```python
from build123d import *

# Parameters (mm, degrees)
SKETCH1_W               = 11.9
SKETCH1_H               = 11.9
BOSS_EXTRUDE1_DEPTH     = 3
CHAMFER1_SIZE           = 0.5
SKETCH3_R               = 3.35
BOSS_EXTRUDE2_DEPTH     = 2
SKETCH4_R               = 0.65
BOSS_EXTRUDE6_DEPTH     = 0.5
SKETCH6_W               = 0.7
SKETCH6_H               = 0.2
MIRROR2_COPY_1_SKETCH_W = 0.7
MIRROR2_COPY_1_SKETCH_H = 0.2


with BuildPart() as part:
    # Sketch1 → Boss-Extrude1 (new body)
    with BuildSketch(Plane(origin=(0, 0, 0), x_dir=(1, 0, 0), z_dir=(0, 1, 0))):
        Rectangle(SKETCH1_W, SKETCH1_H)
    extrude(amount=BOSS_EXTRUDE1_DEPTH)

    # Chamfer1
    chamfer1_edges = [part.edges().sort_by_distance(p)[0] for p in [
        (5.95, 1.5, 5.95),
        (-5.95, 1.5, 5.95),
        (-5.95, 1.5, -5.95),
        (5.95, 1.5, -5.95),
    ]]
    chamfer(chamfer1_edges, length=CHAMFER1_SIZE)

    # Sketch3 → Boss-Extrude2 (add)
    with BuildSketch(Plane(origin=(0, 3, 0), x_dir=(1, 0, 0), z_dir=(0, 1, 0))):
        with Locations(Location((0, 0, 0), (0, 0, 90))):
            Circle(SKETCH3_R)
    extrude(amount=BOSS_EXTRUDE2_DEPTH)

    # Sketch4 → Boss-Extrude6 (add)
    with BuildSketch(Plane(origin=(0, 3, 0), x_dir=(1, 0, 0), z_dir=(0, 1, 0))):
        with Locations(Location((4.2, 4.2, 0), (0, 0, 90))):
            Circle(SKETCH4_R)
        with Locations(Location((4.2, -4.2, 0), (0, 0, 90))):
            Circle(SKETCH4_R)
        with Locations(Location((-4.2, 4.2, 0), (0, 0, 90))):
            Circle(SKETCH4_R)
        with Locations(Location((-4.2, -4.2, 0), (0, 0, 90))):
            Circle(SKETCH4_R)
    extrude(amount=BOSS_EXTRUDE6_DEPTH)

    # Sweep1: sweep along a path in Sketch7
    with BuildLine(Plane.XY) as sweep1_path:
        Line((-5.95, 0.9), (-6.05, 1.073205081))
        Line((-6.05, 1.073205081), (-6.05, -0.426794919))
        Line((-6.05, -0.426794919), (-5.053614445, -2.152585325))
        Line((-5.053614445, -2.152585325), (-3.25, -3))
        Line((-3.25, -3), (-3.25, -3.5))
    # Sketch6 → Sweep1 (sweep)
    with BuildSketch(Plane.ZY.offset(5.95)):
        with Locations((-4.9, 0.9)):
            Rectangle(SKETCH6_W, SKETCH6_H)
    sweep1 = sweep(path=sweep1_path.line, transition=Transition.RIGHT)

    # Mirror1: Sweep1 across plane
    add(sweep1.mirror(Plane.XY))

    # Mirror2: Sweep1 across plane
    add(sweep1.mirror(Plane(origin=(0, 0, 0), x_dir=(0, 0, 1), z_dir=(1, 0, 0))))

    # Mirror2 copy 1: sweep along a path in Mirror2 copy 1 path
    with BuildLine(Plane(origin=(0, 0, 0), x_dir=(-1, 0, 0), z_dir=(0, 0, -1))) as mirror2_copy_1_path:
        Line((-5.95, 0.9), (-6.05, 1.073205081))
        Line((-6.05, 1.073205081), (-6.05, -0.426794919))
        Line((-6.05, -0.426794919), (-5.053614445, -2.152585325))
        Line((-5.053614445, -2.152585325), (-3.25, -3))
        Line((-3.25, -3), (-3.25, -3.5))
    # Mirror2 copy 1 sketch → Mirror2 copy 1 (sweep)
    with BuildSketch(Plane(origin=(5.95, 0, 0), x_dir=(0, 0, -1), z_dir=(1, 0, 0))):
        with Locations((-4.9, 0.9)):
            Rectangle(MIRROR2_COPY_1_SKETCH_W, MIRROR2_COPY_1_SKETCH_H)
    sweep(path=mirror2_copy_1_path.line, transition=Transition.RIGHT)


solid = part.part
```
Read the model definition and answer for the solid it produces. Units are mm, in the model's axes. A direction names the side the tool comes from. Coordinates: 2 decimals unless noted, no trailing zeros. Write each loop counter-clockwise with the first axis right and the second up, starting at its lowest first coordinate (ties: lowest second). Pieces come first, ordered by that corner, then holes. Notation, with made-up numbers: (-21, 6) - (-6, 6) arc R12 cw to (-6, 21) - close; hole circle Ø1 at (20.5, 24). An arc over 180 degrees is marked (long way). Answer as a JSON object with one key per item and string values. Group by question number.
1. A cutting plane is placed at B-B (x = 0). Determine the outline of the cut face in (y, z), plus the area to 3 significant figures.
2. Consider L1, parallel to Y at x = -1.25, z = 0; L2, parallel to Y at x = 5.5, z = 2.25; L3, parallel to X at y = 2.75, z = 5.25. Determine where each line is inside the solid, lowest interval first. Write a range as [from, to].
3. A cutting plane is placed at A-A (y = 1.75). Determine the outline of the cut face in (x, z).
4. A cutting plane is placed at C-C (x = -4.2). Determine the outline of the cut face in (y, z), plus the area to 3 significant figures.
5. Each of these flat-tipped pins is pushed along its axis until it touches: P1, Ø0.7, axis at x = 4, z = -4, coming from the +Y side; P2, Ø0.9, axis at y = 2, z = 2.5, coming from the -X side; P3, Ø3, axis at x = -4.5, y = -2, coming from the +Z side. Where does it stop, or does it pass through?
6. The mould has two halves that part along X. Classify faces 1 (the flat face through (4, 3.5, 4)), 2 (the flat face through (3, 3, -3)), 3 (the cylindrical face through (2.038, 3.986, 2.658)): +X half, -X half, draft (parallel to the pull), parting line (faces both ways), or undercut.
7. A cutting plane is placed at D-D (z = 4.2). Determine the outline of the cut face in (x, y).
8. Which of the six approach directions +Z, -Z, +X, -X, +Y, -Y give full straight-line access (tool end or side, diameter ignored) to faces 4 (the flat face through (-4, 3.5, -4)), 5 (the cylindrical face through (-3.623, 3.246, 3.9))?
Worked out:
{
 "1": {"outline": "(0, -5.95) - (3, -5.95) - (3, -3.35) - (5, -3.35) - (5, 3.35) - (3, 3.35) - (3, 5.95) - (0, 5.95) - close", "area": "49.1 mm²"},
 "2": {"L1": "y = [0, 5]", "L2": "y = [0, 3]", "L3": "x = [-5.95, 5.95]"},
 "3": {"outline": "(-5.95, -5.45) - (-5.45, -5.95) - (5.45, -5.95) - (5.95, -5.45) - (5.95, 5.45) - (5.45, 5.95) - (-5.45, 5.95) - (-5.95, 5.45) - close"},
 "4": {"outline": "(-2.61, -5.25) - (-2.5, -5.25) - (-2.5, -4.55) - (-2.61, -4.55) - close; (-2.61, 4.55) - (-2.5, 4.55) - (-2.5, 5.25) - (-2.61, 5.25) - close; (0, -5.95) - (3, -5.95) - (3, -4.85) - (3.5, -4.85) - (3.5, -3.55) - (3, -3.55) - (3, 3.55) - (3.5, 3.55) - (3.5, 4.85) - (3, 4.85) - (3, 5.95) - (0, 5.95) - close", "area": "37.2 mm²"},
 "5": {"P1": "stops at y = 3.5", "P2": "stops at x = -5.95", "P3": "stops at z = 5.25"},
 "6": {"face 1": "draft", "face 2": "undercut", "face 3": "parting line"},
 "7": {"outline": "(-5.95, 0) - (5.95, 0) - (5.95, 3) - (4.85, 3) - (4.85, 3.5) - (3.55, 3.5) - (3.55, 3) - (-3.55, 3) - (-3.55, 3.5) - (-4.85, 3.5) - (-4.85, 3) - (-5.95, 3) - close"},
 "8": {"face 4": "+Z, -Z, +X, -X, +Y", "face 5": "+Y"}
}
